Can you work these out from the model? Positions are in its coordinate system, mm. Coordinates: 2 decimals unless noted, no trailing zeros. Order: outer loops, then holes, each group sorted by start corner. A loop starts at its lowest first (then second) coordinate and runs counter-clockwise, first axis right, second up. Notation, with made-up numbers: (53.25, -34) -> (62.25, -34) arc R31 ccw to (62.25, -4) -> close; hole circle Ø6 at (5.5, 22.5). An arc over 180 degrees is marked (long way). Answer as CSV lines item,"result".
Autodesk Inventor part; units mm, degrees
ref_plane "YZ Plane" through (0, 0, 0) normal (1, 0, 0) x (0, 1, 0)
ref_plane "XZ Plane" through (0, 0, 0) normal (0, 1, 0) x (-1, 0, 0)
ref_plane "XY Plane" through (0, 0, 0) normal (0, 0, 1) x (1, 0, 0)
sketch "Sketch1" plane through (0, 0, 0) normal (0, 0, 1) x (1, 0, 0)
  line L0 (-25, 0) -> (25, 0)
  line L1 (25, 0) -> (25, 350)
  line L2 (25, 350) -> (-25, 350)
  line L3 (-25, 350) -> (-25, 0)
  circle A0 centre (0, 100.214) radius 6.35
  circle A1 centre (0, 310) radius 6.35
  circle A2 centre (-12.5, 26.5) radius 3.25
  circle A3 centre (12.5, 26.5) radius 3.25
  point P0 (0, 0)
  dimension "d0" = 50
  dimension "d1" = 350
  dimension "d2" = 12.7
  dimension "d3" = 12.7
  dimension "d4" = 6.5
  dimension "d5" = 6.5
extrude "Extrusion1" add sketch "Sketch1" along normal blind 6.5
sketch "Sketch2" plane through (0, 0, 6.5) normal (0, 0, 1) x (1, 0, 0)
  point P0 (0, 0)
properties part number "Main Support"
Q1. Imagine slicing it at C-C (y = 26.5). List the corners of the cut face in (x, z) for me, and give its area (4 significant figures).
Solution:
outline,"(-25, 0) -> (-15.75, 0) -> (-15.75, 6.5) -> (-25, 6.5) -> close; (-9.25, 0) -> (9.25, 0) -> (9.25, 6.5) -> (-9.25, 6.5) -> close; (15.75, 0) -> (25, 0) -> (25, 6.5) -> (15.75, 6.5) -> close"
area,"240.5 mm2"
Q2. If I drill on line 1 (X direction, y = 310, z = 2.5); line 2 (Y direction, x = -12.5, z = 2.5); line 3 (Y direction, x = 15.5, z = 0.5), over which ranges is the centre line in solid material (lowest first)?
Solution:
line 1,"-25 to -6.35, 6.35 to 25"
line 2,"0 to 23.25, 29.75 to 350"
line 3,"0 to 25.25, 27.75 to 350"
Q3. Imagine slicing it at D-D (x = 0). List the corners of the cut face in (y, z) for me.
Solution:
outline,"(0, 0) -> (93.86, 0) -> (93.86, 6.5) -> (0, 6.5) -> close; (106.56, 0) -> (303.65, 0) -> (303.65, 6.5) -> (106.56, 6.5) -> close; (316.35, 0) -> (350, 0) -> (350, 6.5) -> (316.35, 6.5) -> close"
Q4. We'd pull the mould along Y, two halves only. Please class faces 1 (the flat face through (0, 350, 3)), 2 (the cylindrical face through (-1.377, 106.413, 3.204)), 3 (the flat face through (25, 173, 3)): pulls with the +Y half, pulls with the -Y half, needs draft (parallel to the pull), parting line crosses it, or undercut.
Solution:
face 1,"pulls with the +Y half"
face 2,"undercut"
face 3,"needs draft"
Q5. Imagine slicing it at B-B (y = 310). List the corners of the cut face in (x, z) for me, and give its area (3 significant figures).
Solution:
outline,"(-25, 0) -> (-6.35, 0) -> (-6.35, 6.5) -> (-25, 6.5) -> close; (6.35, 0) -> (25, 0) -> (25, 6.5) -> (6.35, 6.5) -> close"
area,"242 mm2"
Q6. Imagine slicing it at A-A (x = -12.5). List the corners of the cut face in (y, z) for me, and give its area (3 significant figures).
Solution:
outline,"(0, 0) -> (23.25, 0) -> (23.25, 6.5) -> (0, 6.5) -> close; (29.75, 0) -> (350, 0) -> (350, 6.5) -> (29.75, 6.5) -> close"
area,"2,230 mm2"
